Design review of the part built by this model. Coordinates are the model's own, in mm. A direction names the side the tool comes from. Give positions to 0.01 mm unless a question says otherwise; leave off trailing zeros. Write each loop counter-clockwise with the first axis right and the second up, starting at its lowest first coordinate (ties: lowest second). Pieces come first, ordered by that corner, then holes. Notation, with made-up numbers: (69.25, 57) - (73.25, 57) arc R16 cw to (73.25, 62) - close; hole circle Ø2 at (28.25, 58). An arc over 180 degrees is marked (long way). Use a Markdown table: item, result. Add a question column.
```python
from build123d import *

# Parameters (mm, degrees)
SKETCH1_W           = 31
SKETCH1_H           = 12.8
BOSS_EXTRUDE1_DEPTH = 0.5
SKETCH2_R           = 1.525
CUT_EXTRUDE1_DEPTH  = 17.799107119
BOSS_EXTRUDE5_DEPTH = 4
BOSS_EXTRUDE3_DEPTH = 3
SKETCH6_R           = 2.2
BOSS_EXTRUDE4_DEPTH = 10.4
CUT_EXTRUDE2_START  = -6.4
CUT_EXTRUDE2_DEPTH  = 6.4
BOSS_EXTRUDE6_START = 3.5
SKETCH12_R          = 1.7
BOSS_EXTRUDE6_DEPTH = 3.5
CHAMFER1_SIZE       = 1
FILLET1_R           = 1
FILLET2_R           = 0.4


with BuildPart() as part:
    # Sketch1 → Boss-Extrude1 (new, symmetric)
    with BuildSketch(Plane.XY):
        Rectangle(SKETCH1_W, SKETCH1_H)
    extrude(amount=BOSS_EXTRUDE1_DEPTH, both=True)

    # Sketch2 → Cut-Extrude1 (cut, through all)
    with BuildSketch(Plane.XY.offset(0.5)):
        with Locations((12.5, 0)):
            Circle(SKETCH2_R)
        with Locations((-12.5, 0)):
            Circle(SKETCH2_R)
    extrude(amount=-CUT_EXTRUDE1_DEPTH, mode=Mode.SUBTRACT)

    # Sketch10 → Boss-Extrude5 (add)
    with BuildSketch(Plane.XY.offset(0.5)):
        with BuildLine():
            Line((-7.526189367, -3.287698228), (-8.526189367, 2.712301772))
            ThreePointArc((-8.526189367, 2.712301772), (-8.135284969, 4.131156068), (-6.8, 4.75))
            Line((-6.8, 4.75), (6.8, 4.75))
            ThreePointArc((6.8, 4.75), (8.135284969, 4.131156068), (8.526189367, 2.712301772))
            Line((8.526189367, 2.712301772), (7.526189367, -3.287698228))
            ThreePointArc((7.526189367, -3.287698228), (6.931156068, -4.335284969), (5.8, -4.75))
            Line((5.8, -4.75), (-5.8, -4.75))
            ThreePointArc((-5.8, -4.75), (-6.931156068, -4.335284969), (-7.526189367, -3.287698228))
        make_face()
        with BuildLine():
            Line((-7.032992405, -3.205498734), (-8.032992405, 2.794501266))
            ThreePointArc((-8.032992405, 2.794501266), (-7.753774978, 3.80796862), (-6.8, 4.25))
            Line((-6.8, 4.25), (6.8, 4.25))
            ThreePointArc((6.8, 4.25), (7.753774978, 3.80796862), (8.032992405, 2.794501266))
            Line((8.032992405, 2.794501266), (7.032992405, -3.205498734))
            ThreePointArc((7.032992405, -3.205498734), (6.60796862, -3.953774978), (5.8, -4.25))
            Line((5.8, -4.25), (-5.8, -4.25))
            ThreePointArc((-5.8, -4.25), (-6.60796862, -3.953774978), (-7.032992405, -3.205498734))
        make_face(mode=Mode.SUBTRACT)
    extrude(amount=BOSS_EXTRUDE5_DEPTH)

    # Sketch5 → Boss-Extrude3 (add)
    with BuildSketch(Plane(origin=(0, 0, -0.5), x_dir=(-1, 0, 0), z_dir=(0, 0, -1))):
        with BuildLine():
            Line((8.019386329, -3.369897721), (9.019386329, 2.630102279))
            ThreePointArc((9.019386329, 2.630102279), (8.516794961, 4.454343516), (6.8, 5.25))
            Line((6.8, 5.25), (-6.8, 5.25))
            ThreePointArc((-6.8, 5.25), (-8.516794961, 4.454343516), (-9.019386329, 2.630102279))
            Line((-9.019386329, 2.630102279), (-8.019386329, -3.369897721))
            ThreePointArc((-8.019386329, -3.369897721), (-7.254343516, -4.716794961), (-5.8, -5.25))
            Line((-5.8, -5.25), (5.8, -5.25))
            ThreePointArc((5.8, -5.25), (7.254343516, -4.716794961), (8.019386329, -3.369897721))
        make_face()
    extrude(amount=BOSS_EXTRUDE3_DEPTH)

    # Sketch6 → Boss-Extrude4 (add)
    with BuildSketch(Plane(origin=(0, 0, -3.5), x_dir=(-1, 0, 0), z_dir=(0, 0, -1))):
        with Locations((-3.4, 0)):
            Circle(SKETCH6_R)
        with Locations(Location((3.4, 0, 0), (0, 0, 180))):
            Circle(SKETCH6_R)
    extrude(amount=BOSS_EXTRUDE4_DEPTH)

    # Sketch7 → Cut-Extrude2 (cut)
    with BuildSketch(Plane(origin=(0, 0, -13.9), x_dir=(-1, 0, 0), z_dir=(0, 0, -1)).offset(CUT_EXTRUDE2_START)):
        with BuildLine():
            Line((-5.1, 0), (-5.1, 1.396424004))
            ThreePointArc((-5.1, 1.396424004), (-3.4, 2.2), (-1.7, 1.396424004))
            Line((-1.7, 1.396424004), (-1.7, 0))
            ThreePointArc((-1.7, 0), (-3.4, -1.7), (-5.1, 0))
        make_face()
        with BuildLine():
            Line((1.7, 0), (1.7, 1.396424004))
            ThreePointArc((1.7, 1.396424004), (3.4, 2.2), (5.1, 1.396424004))
            Line((5.1, 1.396424004), (5.1, 0))
            ThreePointArc((5.1, 0), (3.4, -1.7), (1.7, 0))
        make_face()
    extrude(amount=CUT_EXTRUDE2_DEPTH, mode=Mode.SUBTRACT)

    # Sketch12 → Boss-Extrude6 (add)
    with BuildSketch(Plane.XY.offset(0.5).offset(BOSS_EXTRUDE6_START)):
        with Locations((-3.4, 0)):
            Circle(SKETCH12_R)
        with Locations((3.4, 0)):
            Circle(SKETCH12_R)
    extrude(amount=-BOSS_EXTRUDE6_DEPTH)

    # Chamfer1
    chamfer1_edges = [part.edges().sort_by_distance(p)[0] for p in [
        (-5.1, 0, 4),
        (1.7, 0, 4),
    ]]
    chamfer(chamfer1_edges, length=CHAMFER1_SIZE)

    # Fillet1
    fillet1_edges = [part.edges().sort_by_distance(p)[0] for p in [
        (-15.5, 6.4, 0),
        (15.5, 6.4, 0),
        (15.5, -6.4, 0),
        (-15.5, -6.4, 0),
    ]]
    fillet(fillet1_edges, radius=FILLET1_R)

    # Fillet2
    fillet2_edges = [part.edges().sort_by_distance(p)[0] for p in [
        (-8.516794961, 4.454343516, -3.5),
        (0, 5.25, -3.5),
        (8.516794961, 4.454343516, -3.5),
        (8.519386329, -0.369897721, -3.5),
        (7.254343516, -4.716794961, -3.5),
        (0, -5.25, -3.5),
        (-7.254343516, -4.716794961, -3.5),
        (-8.519386329, -0.369897721, -3.5),
    ]]
    fillet(fillet2_edges, radius=FILLET2_R)


solid = part.part
```
(1) Tool access review of faces 1 (the face through (-8.02, -0.33, 2.47)), 2 (the face through (0, 4.25, 2)), 3 (the face through (7.271, -4.702, -1.782)): name each direction out of +Z, -Z, +X, -X, +Y, -Y from which nothing blocks a thin tool from reaching the whole face with its end or side.
(2) For line 1 along X through (y, z) = (0.75, -8); line 2 along X through (y, z) = (-0.75, -10.75); line 3 along Y through (x, z) = (-12.5, 0.35) (3 decimals), list the stretches that pass through material, from the lowest coordinate up.
(3) Add section A-A (x = 12.5). State the section outline as (y, z) points (3 decimals).
(4) Add section D-D (z = -4). State the section outline as (x, y) points.
(5) Insertion check: pin 1 (1.5 mm diameter, centred on y = 2, z = -11, fed in from +X); pin 2 (1.3 mm diameter, centred on x = -1.5, z = -1.5, fed in from -Y); pin 3 (2 mm diameter, centred on x = -0.5, z = 2.5, fed in from +Y). Each pin has a flat end and moves straight along its axis. Give the tip position at first contact, or say it passes through.
(6) Mouldability with a two-part tool opening along X and no side actions: class faces 4 (the face through (0, -6, -0.5)), 5 (the face through (-3.4, -1.7, -10.7)), 6 (the face through (8.526, -0.328, -1.782)) as +X half, -X half, draft (parallel to the pull), parting line (faces both ways), or undercut.
(7) Add section B-B (z = -8.75). State the section outline as (x, y) points, and give its area (3 significant figures).
Answers follow:
| question | item | result |
|---|---|---|
| 1 | face 1 | +Z, -X, -Y |
| 1 | face 2 | +Z |
| 1 | face 3 | -Z, +X, -Y |
| 2 | line 1 | -5.47 to -5.1, -1.7 to -1.33, 1.33 to 1.7, 5.1 to 5.47 |
| 2 | line 2 | -5.47 to -4.93, -1.87 to -1.33, 1.33 to 1.87, 4.93 to 5.47 |
| 2 | line 3 | -6.4 to -1.525, 1.525 to 6.4 |
| 3 | outline | (-6.4, -0.5) - (-1.525, -0.5) - (-1.525, 0.5) - (-6.4, 0.5) - close; (1.525, -0.5) - (6.4, -0.5) - (6.4, 0.5) - (1.525, 0.5) - close |
| 4 | outline | circle Ø4.4 at (-3.4, 0); circle Ø4.4 at (3.4, 0) |
| 5 | pin 1 | x = 5.21 |
| 5 | pin 2 | y = -5.25 |
| 5 | pin 3 | y = 4.75 |
| 6 | face 4 | draft |
| 6 | face 5 | undercut |
| 6 | face 6 | +X half |
| 7 | outline | (-5.1, 0) - (-5.1, 1.4) arc R2.2 ccw (long way) to (-1.7, 1.4) - (-1.7, 0) arc R1.7 cw to start; (1.7, 0) - (1.7, 1.4) arc R2.2 ccw (long way) to (5.1, 1.4) - (5.1, 0) arc R1.7 cw to start |
| 7 | area | 8.03 mm^2 |
